For this review, take the finished solid that the model builds, in its own axes (mm). Give positions to 0.01 mm unless a question says otherwise; leave off trailing zeros. Loops run counter-clockwise (first coordinate to the right, second up) from the corner with the lowest first, then second, coordinate; pieces in that order, holes last.
Autodesk Inventor part; units mm, degrees
ref_plane "YZ Plane" through (0, 0, 0) normal (1, 0, 0) x (0, 1, 0)
ref_plane "XZ Plane" through (0, 0, 0) normal (0, 1, 0) x (-1, 0, 0)
ref_plane "XY Plane" through (0, 0, 0) normal (0, 0, 1) x (1, 0, 0)
sketch "Sketch1" plane through (0, 0, 0) normal (0, 1, 0) x (-1, 0, 0)
  line L0 (0, 0) -> (0, -120.239) construction
  line L1 (3, 0) -> (3, -120.239)
  line L2 (-3, -120.239) -> (-3, 0)
  arc A0 (3, 0) -> (-3, 0) centre (0, 0) ccw
  arc A1 (-3, -120.239) -> (3, -120.239) centre (0, -120.239) ccw
  circle A2 centre (0, 0) radius 1.1
  circle A3 centre (0, -120.239) radius 1.1
  arc A4 (-3, -120.239) -> (-3, 0) centre (-296.9144, -60.1195) ccw
  arc A5 (3, -120.239) -> (3, 0) centre (-290.9144, -60.1195) ccw
  point P0 (0, -60.1195)
  dimension "d0" = 2.2
  dimension "d1" = 2.2
  dimension "d2" = 6
  dimension "d3" = 120.239
  dimension "d14" = 300
  dimension "d15" = 300
extrude "Extrusion1" add sketch "Sketch1" along normal blind 4 contours A5 L1 A4 | L1 A4 A0 | A1 A4 L1
Q1. Consider section B-B on x = 0. Give the boundary of the cut face in (y, z).
Answers:
outline: (0, -123.24) - (4, -123.24) - (4, -121.34) - (0, -121.34) - close; (0, -119.14) - (4, -119.14) - (4, -103.04) - (0, -103.04) - close; (0, -17.2) - (4, -17.2) - (4, -1.1) - (0, -1.1) - close; (0, 1.1) - (4, 1.1) - (4, 3) - (0, 3) - close
Q2. Consider section D-D on x = -7.75. Give the boundary of the cut face in (y, z).
Answers:
outline: (0, -88.4) - (4, -88.4) - (4, -31.84) - (0, -31.84) - close
Q3. For probe 1 along X at (y, z) = (0.8, -63); probe 2 along X at (y, z) = (1.7, -33), list the stretches that pass through material, from the lowest coordinate up.
Answers:
probe 1: x = -9.07 to -3.07
probe 2: x = -7.86 to -1.86
Q4. Consider section A-A on y = 1.8. Give the boundary of the cut face in (x, z).
Answers:
outline: (-3, -120.24) arc R3 ccw to (3, -120.24) arc R300 cw to (3, 0) arc R3 ccw to (-3, 0) arc R300 ccw to start; hole circle Ø2.2 at (0, -120.24); hole circle Ø2.2 at (0, 0)
Q5. Consider section C-C on z = -41. Give the boundary of the cut face in (x, y).
Answers:
outline: (-8.48, 0) - (-2.48, 0) - (-2.48, 4) - (-8.48, 4) - close
Q6. Mouldability with a two-part tool opening along X and no side actions: class faces 1 (the flat face through (-4, 0, -59)), 2 (the cylindrical face through (-9.084, 1.972, -59.272)), 3 (the cylindrical face through (-1.05, 1.97, -0.33)) as +X half, -X half, draft (parallel to the pull), parting line (faces both ways), or undercut.
Answers:
face 1: draft
face 2: -X half
face 3: undercut
Q7. For pin 1 Ø2 at (x, z) = (0, 0) entering from +Y; pin 2 Ø1 at (y, z) = (0.5, -31) entering from +X, all flat-tipped, find the tip position at first contact; note any pin that passes through.
Answers:
pin 1: passes through
pin 2: stops at x = -1.62
